Design review of the part shown in the three views and the two pictorial views. Dimensions are in mm from the part's minimum x, y and z. A direction names the side the tool comes from. Coordinates: 2 decimals unless noted, no trailing zeros. Order: outer loops, then holes, each group sorted by start corner. A loop starts at its lowest first (then second) coordinate and runs counter-clockwise, first axis right, second up. Notation, with made-up numbers: (-33, 86) -> (23, 86) arc R17 cw to (23, 110) -> close; hole circle Ø4 at (-30, 59.25). An arc over 180 degrees is marked (long way). Answer as a JSON object with one key per item and string values. Group by question number.
1) For pin 1 (3 mm diameter, centred on x = 71, y = 41, fed in from +Z); pin 2 (22 mm diameter, centred on x = 49.5, z = 35.5, fed in from -Y); pin 3 (17.5 mm diameter, centred on x = 80, z = 31.5, fed in from -Y), all flat-tipped, find the tip position at first contact; note any pin that passes through.
2) Machinability: for the marked faces 4, 5, 6, 7 and 8, which of the approach directions +Z, -Z, +X, -X, +Y, -Y give a long, thin tool a straight path to every point of the face, cutting with its end or side? Answer none if there is none.
3) Wall thickness on L1, parallel to X at y = 49, z = 61; L2, parallel to X at y = 38.5, z = 45; L3, parallel to Y at x = 84, z = 45: over which ranges is each line inside the solid? List them lowest first.
4) Add section D-D, the plane y = 69.5. Write out the cut boundary in (x, z).
5) Draft analysis for pull direction X (two halves, no side actions). For the marked faces 1, 2 and 3, state which applies: +X half, -X half, draft (parallel to the pull), parting line (faces both ways), or undercut.
6) Add section C-C, the plane z = 30. Write out the cut boundary in (x, y).
7) Add section A-A, the plane z = 68.5. Write out the cut boundary in (x, y).
8) Add section B-B, the plane y = 33. Write out the cut boundary in (x, z).
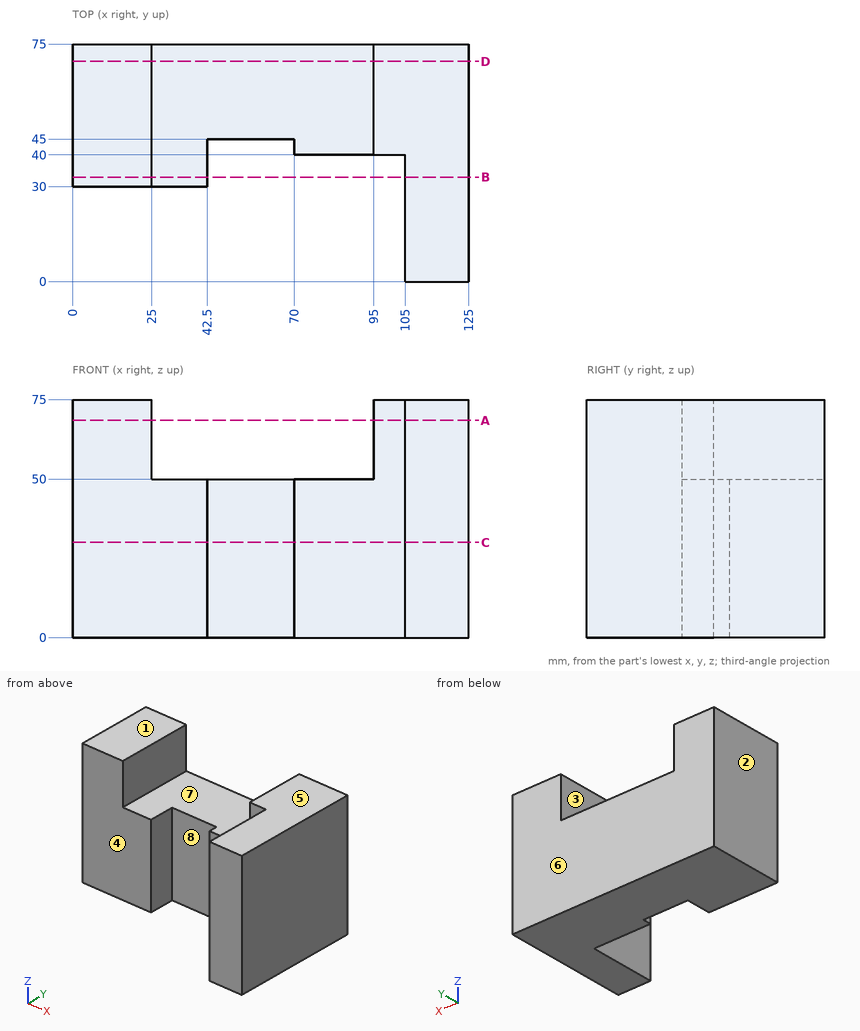
Output values:
{
 "1": {"pin 1": "stops at z = 50", "pin 2": "stops at y = 30", "pin 3": "stops at y = 40"},
 "2": {"face 4": "+Z, -Z, -X, -Y", "face 5": "+Z, +X, -X, +Y, -Y", "face 6": "+Z, -Z, +X, -X, +Y", "face 7": "+Z, +Y, -Y", "face 8": "+Z, -Z, -Y"},
 "3": {"L1": "x = 0 to 25, 95 to 125", "L2": "x = 0 to 42.5, 105 to 125", "L3": "y = 40 to 75"},
 "4": {"outline": "(0, 0) -> (125, 0) -> (125, 75) -> (95, 75) -> (95, 50) -> (25, 50) -> (25, 75) -> (0, 75) -> close"},
 "5": {"face 1": "draft", "face 2": "-X half", "face 3": "undercut"},
 "6": {"outline": "(0, 30) -> (42.5, 30) -> (42.5, 45) -> (70, 45) -> (70, 40) -> (105, 40) -> (105, 0) -> (125, 0) -> (125, 75) -> (0, 75) -> close"},
 "7": {"outline": "(0, 30) -> (25, 30) -> (25, 75) -> (0, 75) -> close; (95, 40) -> (105, 40) -> (105, 0) -> (125, 0) -> (125, 75) -> (95, 75) -> close"},
 "8": {"outline": "(0, 0) -> (42.5, 0) -> (42.5, 50) -> (25, 50) -> (25, 75) -> (0, 75) -> close; (105, 0) -> (125, 0) -> (125, 75) -> (105, 75) -> close"}
}
